```python
from build123d import *

# Parameters (mm, degrees)
CHAFL_N1_SIZE                                  = 0.5
PERFORADOR_PARA_ROSCAR_PARA_MACHO_DE_ROS_D     = 2.5
PERFORADOR_PARA_ROSCAR_PARA_MACHO_DE_ROS_DEPTH = 6
PERFORADOR_PARA_ROSCAR_PARA_MACHO_DE_ROS_TIP   = 0.751075774
CROQUIS12_W                                    = 1.25
CROQUIS12_H                                    = 6
TALADROS_DE_ESPIGA_DE_6_0MM1_D                 = 6
TALADROS_DE_ESPIGA_DE_6_0MM1_DEPTH             = 14
TALADROS_DE_ESPIGA_DE_6_0MM1_TIP               = 1.802581857
PERFORADOR_PARA_ROSCAR_PARA_MACHO_DE_3_D       = 2.5
PERFORADOR_PARA_ROSCAR_PARA_MACHO_DE_3_DEPTH   = 2.248924226
PERFORADOR_PARA_ROSCAR_PARA_MACHO_DE_3_TIP     = 0.751075774


with BuildPart() as part:
    # Croquis1 → Revolución1 (revolve)
    with BuildSketch(Plane(origin=(0, 0, 0), x_dir=(-1, 0, 0), z_dir=(0, 1, 0)), mode=Mode.PRIVATE) as revoluci_n1_sk:
        Polygon((-45.3, 3), (-45.3, 6), (-28.7, 6), (-27.2, 4.5), (-27.2, 3), (25.7, 3), (25.7, 2.55), (26.5, 2.55), (26.5, 3), (30.7, 3), (30.7, 0), (-30.7, 0), (-45.3, 0), align=None)
    revolve(revoluci_n1_sk.sketch.rotate(Axis((30.7, 0, 0), (-1, 0, 0)), 180), axis=Axis((30.7, 0, 0), (-1, 0, 0)))

    # Chaflán1
    chafl_n1_edges = [part.edges().sort_by_distance(p)[0] for p in [
        (-30.7, 0, 3),
    ]]
    chamfer(chafl_n1_edges, length=CHAFL_N1_SIZE)

    # Perforador para roscar para macho de ros
    with Locations(Plane(origin=(0, 6, -6), x_dir=(0, 0, 1), z_dir=(0, 1, 0))):
        with Locations((6, 37.3)):
            Hole(PERFORADOR_PARA_ROSCAR_PARA_MACHO_DE_ROS_D / 2, depth=PERFORADOR_PARA_ROSCAR_PARA_MACHO_DE_ROS_DEPTH)
            with Locations((0, 0, -(PERFORADOR_PARA_ROSCAR_PARA_MACHO_DE_ROS_DEPTH + PERFORADOR_PARA_ROSCAR_PARA_MACHO_DE_ROS_TIP / 2))):  # 118° drill point
                Cone(0, PERFORADOR_PARA_ROSCAR_PARA_MACHO_DE_ROS_D / 2, PERFORADOR_PARA_ROSCAR_PARA_MACHO_DE_ROS_TIP, mode=Mode.SUBTRACT)

    # Croquis12 → Perforador para roscar para macho de 2 (revolve, cut)
    with BuildSketch(Plane.YZ.offset(37.3)):
        with Locations((0.625, 3)):
            Rectangle(CROQUIS12_W, CROQUIS12_H)
    revolve(axis=Axis((37.3, 0, -6.35), (0, 0, 1)), mode=Mode.SUBTRACT)

    # Taladros de espiga de Ø6.0mm1
    with Locations(Plane.YZ.offset(45.3)):
        with Locations((0, 0)):
            Hole(TALADROS_DE_ESPIGA_DE_6_0MM1_D / 2, depth=TALADROS_DE_ESPIGA_DE_6_0MM1_DEPTH)
            with Locations((0, 0, -(TALADROS_DE_ESPIGA_DE_6_0MM1_DEPTH + TALADROS_DE_ESPIGA_DE_6_0MM1_TIP / 2))):  # 118° drill point
                Cone(0, TALADROS_DE_ESPIGA_DE_6_0MM1_D / 2, TALADROS_DE_ESPIGA_DE_6_0MM1_TIP, mode=Mode.SUBTRACT)

    # Perforador para roscar para macho de 3
    with Locations(Plane(origin=(-9.7, 2.417350066, 1.776631267), x_dir=(0, -0.592210422366, 0.805783355276), z_dir=(0, 0.805783355276, 0.592210422366))):
        with Locations((0, 0)):
            Hole(PERFORADOR_PARA_ROSCAR_PARA_MACHO_DE_3_D / 2, depth=PERFORADOR_PARA_ROSCAR_PARA_MACHO_DE_3_DEPTH)
            with Locations((0, 0, -(PERFORADOR_PARA_ROSCAR_PARA_MACHO_DE_3_DEPTH + PERFORADOR_PARA_ROSCAR_PARA_MACHO_DE_3_TIP / 2))):  # 118° drill point
                Cone(0, PERFORADOR_PARA_ROSCAR_PARA_MACHO_DE_3_D / 2, PERFORADOR_PARA_ROSCAR_PARA_MACHO_DE_3_TIP, mode=Mode.SUBTRACT)


solid = part.part
```
Here's how the part is built. I have some questions about the finished solid (model axes, mm). A direction names the side the tool comes from. Give positions to 0.01 mm unless a question says otherwise; leave off trailing zeros. Write each loop counter-clockwise with the first axis right and the second up, starting at its lowest first coordinate (ties: lowest second). Pieces come first, ordered by that corner, then holes. Notation, with made-up numbers: (-5.5, -35) -> (41.5, -35) arc R18 ccw to (41.5, -1) -> close; hole circle Ø11 at (3, -8.5). An arc over 180 degrees is marked (long way). Write each question's results on one line, items separated by ' | '.
Item 1: If I drill on L1, parallel to X at y = 0, z = 3.4; L2, parallel to X at y = -1.5, z = -3; L3, parallel to Z at x = 37.3, y = 4.15, over which ranges is the centre line in solid material (lowest first)?
Output:
L1: x = 27.2 to 36.05, 38.55 to 45.3 | L2: x = 27.2 to 45.3 | L3: z = -4.33 to -1.25, 1.25 to 4.33
Item 2: Suppose I cut it at B-B on x = 5. Write out the boundary of the cut face in (y, z).
Output:
outline: circle Ø6 at (0, 0)
Item 3: We'd pull the mould along Z, two halves only. Please class faces 1 (the face through (-28.38, -0.9, -2.86)), 2 (the face through (-9.325, 2.206, 0.142)), 3 (the face through (-26.5, -2, -2)): pulls with the +Z half, pulls with the -Z half, needs draft (parallel to the pull), parting line crosses it, or undercut.
Output:
face 1: parting line crosses it | face 2: undercut | face 3: needs draft
Item 4: On a 3-axis mill with a long thin cutter (end or side, diameter ignored), from which of +Z, -Z, +X, -X, +Y, -Y can I reach the whole of each face in a straight line? I mean faces 4 (the face through (-9.91, 0.13, 0.04)), 5 (the face through (0.38, -0.9, -2.86)), 6 (the face through (36.06, -0.16, 4.39)). Say none if no direction works.
Output:
face 4: none | face 5: -X | face 6: +Z
Item 5: Suppose I cut it at A-A on x = 37.3. Write out the boundary of the cut face in (y, z).
Output:
outline: (-1.25, 2.73) -> (-1.25, 5.87) arc R6 ccw (long way) to (5.87, -1.25) -> (2.73, -1.25) arc R3 cw (long way) to start; (1.25, 2.73) arc R3 cw to (2.73, 1.25) -> (5.87, 1.25) arc R6 ccw to (1.25, 5.87) -> close
Item 6: For pin 1 Ø1.5 at (x, y) = (30.5, -3) entering from +Z; pin 2 Ø4 at (x, y) = (-2.5, -4.5) entering from -Z; pin 3 Ø3 at (x, z) = (0.5, 3.5) entering from +Y, each with a flat end and sliding along its axis, tell me the tip position at first contact or that it passes through.
Output:
pin 1: stops at z = 5.56 | pin 2: stops at z = -1.66 | pin 3: stops at y = 2.24
